from build123d import *

# Parameters (mm, degrees)
SKETCH_1_R          = 1.9
EXTRUDE_1_DEPTH     = 69
SKETCH_2_R          = 2.5
CUT_EXTRUDE_1_DEPTH = 2.1


with BuildPart() as part:
    # 草图1 → 凸台-拉伸1 (new body)
    with BuildSketch(Plane(origin=(0, 0, 0), x_dir=(0, 0, -1), z_dir=(1, 0, 0))):
        with Locations((22, 3)):
            Circle(SKETCH_1_R)
        with BuildLine():
            Line((0, 1.1), (0, 0))
            Line((0, 0), (19, 0))
            Line((19, 0), (23.9, 0))
            Line((23.9, 0), (23.9, 3))
            ThreePointArc((23.9, 3), (23.343502884, 1.656497116), (22, 1.1))
            Line((22, 1.1), (19, 1.1))
            Line((19, 1.1), (0, 1.1))
        make_face()
    extrude(amount=EXTRUDE_1_DEPTH)

    # 草图2 → 切除-拉伸1 (cut, through all)
    with BuildSketch(Plane(origin=(0, 1.1, 0), x_dir=(1, 0, 0), z_dir=(0, 1, 0))):
        with Locations((8.5, 10)):
            Circle(SKETCH_2_R)
        with Locations((60.5, 10)):
            Circle(SKETCH_2_R)
        with Locations((34.5, 8)):
            Circle(SKETCH_2_R)
    extrude(amount=-CUT_EXTRUDE_1_DEPTH, mode=Mode.SUBTRACT)


solid = part.part
Geometry check sheet. Reference: the model listing, model coordinates, mm. Coordinates: 2 decimals unless noted, no trailing zeros. Order: outer loops, then holes, each group sorted by start corner. A loop starts at its lowest first (then second) coordinate and runs counter-clockwise, first axis right, second up. Notation, with made-up numbers: (54, 27.5) -> (88, 27.5) arc R4 cw to (88, 33.5) -> close; hole circle Ø7 at (56.5, 8.25). An arc over 180 degrees is marked (long way). Use a Markdown table: item, result. Add a question column.
1. Mould release check, pull along X, two halves, no side actions. Record for faces 1 (the face through (36.81, 0.56, -7.04)), 2 (the face through (7.96, 0.56, -7.56)), 3 (the face through (34, 0.6, 0)), 4 (the face through (0, 0.8, -15.4)): pulls with the +X half, pulls with the -X half, needs draft (parallel to the pull), parting line crosses it, or undercut.
2. Cross-section at A-A (x = 34.5). Enter the section's corners in (y, z).
3. Material ranges on L1, parallel to Z at x = 60.5, y = 0.75; L2, parallel to X at y = 0.9, z = -10; L3, parallel to Z at x = 38, y = 3, recorded low to high.
4. Cross-section at C-C (z = -17.5). Enter the section's corners in (x, y).
5. Go/stop test with flat-tipped pins: pin 1 Ø1 at (x, y) = (20.5, 2.5) entering from +Z; pin 2 Ø6.5 at (x, z) = (8.5, -10) entering from +Y. Record where each tip stops, or that it passes through.
6. Cross-section at B-B (x = 13.5). Enter the section's corners in (y, z), and give its area (3 significant figures).
Filled sheet:
| question | item | result |
|---|---|---|
| 1 | face 1 | undercut |
| 1 | face 2 | undercut |
| 1 | face 3 | needs draft |
| 1 | face 4 | pulls with the -X half |
| 2 | outline | (0, -23.9) -> (3, -23.9) arc R1.9 ccw (long way) to (1.1, -22) -> (1.1, -10.5) -> (0, -10.5) -> close; (0, -5.5) -> (1.1, -5.5) -> (1.1, 0) -> (0, 0) -> close |
| 3 | L1 | -23.9 to -12.5, -7.5 to 0 |
| 3 | L2 | 0 to 6, 11 to 33, 36 to 58, 63 to 69 |
| 3 | L3 | -23.9 to -20.1 |
| 4 | outline | (0, 0) -> (69, 0) -> (69, 1.1) -> (0, 1.1) -> close |
| 5 | pin 1 | z = -20.1 |
| 5 | pin 2 | y = 1.1 |
| 6 | outline | (0, -23.9) -> (3, -23.9) arc R1.9 ccw (long way) to (1.1, -22) -> (1.1, 0) -> (0, 0) -> close |
| 6 | area | 38.4 mm2 |
